CAD build for the part. Positions are in the model's coordinates, mm. Coordinates: 2 decimals unless noted, no trailing zeros. Loops run counter-clockwise (first coordinate to the right, second up) from the corner with the lowest first, then second, coordinate; pieces in that order, holes last. Notation, with made-up numbers: (68.5, -25) -> (110.5, -25) arc R24 cw to (110.5, 12) -> close; hole circle Ø3 at (15, 14.5). An arc over 180 degrees is marked (long way). Return JSON: item names as keys, results as strings. Group by question number.
(1) Probe L1, parallel to Z at x = -122, y = 77; L2, parallel to Z at x = -198, y = 49; L3, parallel to Y at x = -91, z = -39.5. List the from-to ranges inside material, lowest first.
(2) Saw through at A-A on x = -105. Write the cut outline in (y, z).
(3) Saw through at C-C on z = -121.5. Write the cut outline in (x, y), then the cut area to 3 significant figures.
(4) Flat gauge pin, fed straight in: pin 1 Ø8 at (x, y) = (-177.5, 75) entering from +Z. Where does the tip first touch, or does it go through?
(5) Saw through at D-D on x = -55. Write the cut outline in (y, z).
(6) Saw through at B-B on y = 57. Write the cut outline in (x, z).
Autodesk Inventor part; units mm, degrees
ref_plane "YZ Plane" through (0, 0, 0) normal (1, 0, 0) x (0, 1, 0)
ref_plane "XZ Plane" through (0, 0, 0) normal (0, 1, 0) x (-1, 0, 0)
ref_plane "XY Plane" through (0, 0, 0) normal (0, 0, 1) x (1, 0, 0)
sketch "Sketch4" plane through (0, 0, 0) normal (0, 1, 0) x (-1, 0, 0)
  line L0 (0, 0) -> (210, 0)
  line L1 (210, 0) -> (210, -310)
  line L2 (210, -310) -> (0, -310)
  line L3 (0, -310) -> (0, 0)
  dimension "d9" = 310
  dimension "d10" = 210
extrude "Extrusion3" add sketch "Sketch4" along normal blind 150
shell "Shell1" thickness 5 removed faces 0
sketch "Sketch5" plane through (-205, 5, -305) normal (1, 0, 0) x (0, 0, -1)
  line L0 (0, 0) -> (-300, 0)
  line L1 (-214.5126, 0) -> (-209.5126, 0)
  line L2 (-209.5126, 0) -> (-209.5126, 135)
  line L3 (-209.5126, 135) -> (-214.5126, 135)
  line L4 (-214.5126, 135) -> (-214.5126, 0)
  point P0 (-305, -5)
  point P1 (-209.5126, 0)
  dimension "d18" = 5
  dimension "d19" = 135
extrude "Extrusion4" add sketch "Sketch5" along normal blind 200
sketch "Sketch6" plane through (-205, 5, -95.4874) normal (0, 0, -1) x (-1, 0, 0)
  circle A0 centre (-150, 105) radius 5
  circle A1 centre (-100, 105) radius 8.9
  circle A2 centre (-50, 105) radius 5
  line L0 (0, 135) -> (0, 0)
  line L1 (0, 135) -> (-200, 135)
  point P0 (-205, -5)
chamfer "Chamfer1" distance 1 angle 45 4 edges at (-210, 75, -310) (0, 75, -310) (0, 75, 0) (-210, 75, 0)
extrude "Extrusion5" cut sketch "Sketch6" against normal blind 10
sketch "Sketch7" plane through (-205, 5, -5) normal (0, 1, 0) x (1, 0, 0)
  circle A0 centre (7, 7) radius 4
  circle A1 centre (7, 78.4874) radius 4
  circle A2 centre (193, 7) radius 4
  circle A3 centre (193, 78.4874) radius 4
  line L0 (0, 0) -> (200, 0)
  line L1 (200, 0) -> (200, 85.4874)
  line L2 (0, 85.4874) -> (200, 85.4874)
  line L3 (0, 85.4874) -> (0, 0)
  point P0 (205, -5)
  dimension "d37" = 8
  dimension "d38" = 8
  dimension "d39" = 8
  dimension "d40" = 8
  dimension "d41" = 7
  dimension "d42" = 7
  dimension "d43" = 7
  dimension "d44" = 7
  dimension "d45" = 7
  dimension "d46" = 7
  dimension "d47" = 7
  dimension "d48" = 7
extrude "Extrusion6" add sketch "Sketch7" along normal blind 130 contours A0 | A1 | A2 | A3
sketch "Sketch8" plane through (-198, 135, -12) normal (0, 1, 0) x (1, 0, 0)
  circle A0 centre (0, 0) radius 1.5
  circle A1 centre (0, 71.4874) radius 4
  circle A2 centre (0, 71.4874) radius 1.5
  circle A3 centre (186, 0) radius 4
  circle A4 centre (186, 0) radius 1.5
  circle A5 centre (186, 71.4874) radius 4
  circle A6 centre (186, 71.4874) radius 1.5
  point P0 (198, -12)
  dimension "d51" = 3
  dimension "d52" = 3
  dimension "d53" = 3
  dimension "d54" = 3
extrude "Extrusion7" cut sketch "Sketch8" against normal blind 30 contours A0 | A2 | A4 | A6
equation "\"d9\" = Panjang_outer"
equation "\"d10\" = Lebar_outer"
equation "\"d11\" = Tinggi_Box"
equation "\"d42\" = d41"
equation "\"d43\" = d41"
equation "\"d44\" = d41"
equation "\"d45\" = d41"
equation "\"d46\" = d41"
equation "\"d47\" = d41"
equation "\"d48\" = d41"
equation "\"Lebar_outer\" = 210"
equation "\"Panjang_outer\" = 310"
equation "\"Tinggi_Box\" = 150"
properties part number "Box"
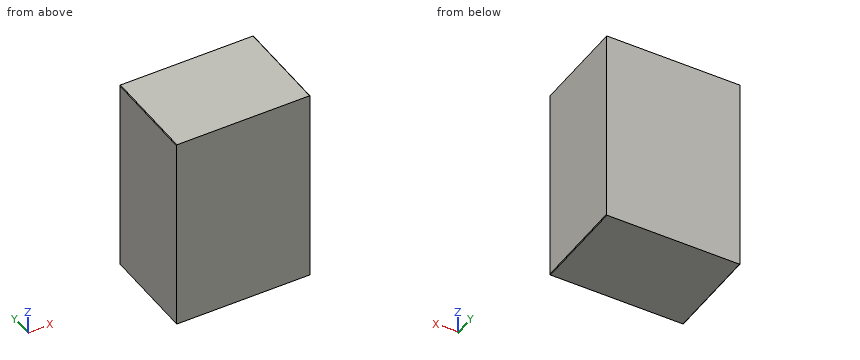
Geometry results:
{
 "1": {"L1": "-310 to -305, -95.49 to -90.49, -5 to 0", "L2": "-310 to -305, -95.49 to -90.49, -87.49 to -79.49, -16 to -8, -5 to 0", "L3": "0 to 5, 145 to 150"},
 "2": {"outline": "(0, -310) -> (150, -310) -> (150, 0) -> (0, 0) -> close; (118.9, -95.49) -> (140, -95.49) -> (140, -90.49) -> (118.9, -90.49) -> close; hole (5, -305) -> (145, -305) -> (145, -5) -> (5, -5) -> (5, -90.49) -> (101.1, -90.49) -> (101.1, -95.49) -> (5, -95.49) -> close"},
 "3": {"outline": "(-210, 0) -> (0, 0) -> (0, 150) -> (-210, 150) -> close; hole (-205, 5) -> (-5, 5) -> (-5, 145) -> (-205, 145) -> close", "area": "3,500 mm²"},
 "4": {"pin 1": "z = 0"},
 "5": {"outline": "(0, -310) -> (150, -310) -> (150, 0) -> (0, 0) -> close; (115, -95.49) -> (140, -95.49) -> (140, -90.49) -> (115, -90.49) -> close; hole (5, -305) -> (145, -305) -> (145, -5) -> (5, -5) -> (5, -90.49) -> (105, -90.49) -> (105, -95.49) -> (5, -95.49) -> close"},
 "6": {"outline": "(-210, -309) -> (-209, -310) -> (-1, -310) -> (0, -309) -> (0, -1) -> (-1, 0) -> (-209, 0) -> (-210, -1) -> close; circle Ø8 at (-198, -83.49); circle Ø8 at (-198, -12); circle Ø8 at (-12, -83.49); circle Ø8 at (-12, -12); hole (-205, -305) -> (-5, -305) -> (-5, -95.49) -> (-205, -95.49) -> close; hole (-205, -90.49) -> (-5, -90.49) -> (-5, -5) -> (-205, -5) -> close"}
}
